from build123d import *

# Parameters (mm, degrees)
CUT_EXTRUDE1_DEPTH      = 136.830777072
CUT_EXTRUDE1_DEPTH_BACK = 136.830777072
SKETCH2_R               = 6
CUT_EXTRUDE2_DEPTH      = 91.967026993
CUT_EXTRUDE2_DEPTH_BACK = 91.967026993
SKETCH4_R               = 2.5


with BuildPart() as part:
    # Sketch1 → Revolve1 (revolve)
    with BuildSketch(Plane(origin=(0, 0, 0), x_dir=(0, 0, -1), z_dir=(1, 0, 0))):
        with BuildLine():
            Line((-42.5, 55), (-42.5, -52.5))
            ThreePointArc((-42.5, -52.5), (-39.571067812, -59.571067812), (-32.5, -62.5))
            Line((-32.5, -62.5), (0, -62.5))
            Line((0, -62.5), (0, -65))
            Line((0, -65), (-35, -65))
            ThreePointArc((-35, -65), (-42.071067812, -62.071067812), (-45, -55))
            Line((-45, -55), (-45, 55))
            Line((-45, 55), (-42.5, 55))
        make_face()
    revolve(axis=Axis((0, 51.85854301, 0), (0, -1, 0)))

    # Sketch2 → Cut-Extrude1 (cut, two sides: drawn at the far end of the back side and taken through both)
    with BuildSketch(Plane.XZ.offset(65).offset(-CUT_EXTRUDE1_DEPTH_BACK)):
        with Locations(Location((0, 12.5, 0), (0, 0, 270))):
            Circle(SKETCH2_R)
        with Locations(Location((0, -12.5, 0), (0, 0, 270))):
            Circle(SKETCH2_R)
    extrude(amount=CUT_EXTRUDE1_DEPTH + CUT_EXTRUDE1_DEPTH_BACK, mode=Mode.SUBTRACT)

    # Sketch4 → Cut-Extrude2 (cut, two sides: drawn at the far end of the back side and taken through both)
    with BuildSketch(Plane.XY.offset(-CUT_EXTRUDE2_DEPTH_BACK)):
        with Locations(Location((0, -5, 0), (0, 0, 180))):
            Circle(SKETCH4_R)
        with Locations(Location((0, -35, 0), (0, 0, 180))):
            Circle(SKETCH4_R)
    extrude(amount=CUT_EXTRUDE2_DEPTH + CUT_EXTRUDE2_DEPTH_BACK, mode=Mode.SUBTRACT)


solid = part.part
Here's how the part is built. I have some questions about the finished solid (model axes, mm). A direction names the side the tool comes from. Give positions to 0.01 mm unless a question says otherwise; leave off trailing zeros. Order: outer loops, then holes, each group sorted by start corner. A loop starts at its lowest first (then second) coordinate and runs counter-clockwise, first axis right, second up. Notation, with made-up numbers: (58.25, 41) -> (77.25, 41) arc R25 cw to (77.25, 73) -> close; hole circle Ø10 at (70, 39). An arc over 180 degrees is marked (long way). Use a Markdown table: item, result. Add a question column.
Item 1: I need wall thicknesses on line 1 (Z direction, x = 0, y = -22); line 2 (Y direction, x = 0, z = -43.8); line 3 (Y direction, x = 0, z = -43.65). Which ranges of each line are inside material? Lowest first, please.
Item 2: If we mould it in two halves opening along Z, with no side actions, what happens to faces 1 (the face through (0.33, -7.48, 43.7)), 2 (the face through (-2.3, -63.73, -18.04)), 3 (the face through (17.235, 0.77, 41.569))? For each: pulls with the +Z half, pulls with the -Z half, needs draft (parallel to the pull), parting line crosses it, or undercut.
Item 3: Imagine slicing it at C-C on y = -47. Please give me the cut outline in (x, z).
Item 4: Imagine slicing it at B-B on z = 0. Please give me the cut outline in (x, y), plus the area to 4 significant figures.
Item 5: Will these pins go through, and if not, where does the flat tip stop? pin 1 (5 mm diameter, centred on x = 10.5, z = -28, fed in from +Y); pin 2 (2 mm diameter, centred on y = -16.5, z = -31, fed in from +X); pin 3 (11 mm diameter, centred on x = 0, z = 12.5, fed in from +Y); pin 4 (5 mm diameter, centred on y = -4.5, z = 21, fed in from +X).
Item 6: For faces 4 (the face through (0.54, -32.56, -43.73)), 5 (the face through (0, -62.5, 0)), which set-ups out of +Z, -Z, +X, -X, +Y, -Y let a thin tool reach every point of the face, with its end or its side?
Data:
| question | item | result |
|---|---|---|
| 1 | line 1 | z = -45 to -42.5, 42.5 to 45 |
| 1 | line 2 | y = -59.75 to -37.5, -32.5 to -7.5, -2.5 to 55 |
| 1 | line 3 | y = -60.02 to -37.5, -32.5 to -7.5, -2.5 to 55 |
| 2 | face 1 | needs draft |
| 2 | face 2 | undercut |
| 2 | face 3 | parting line crosses it |
| 3 | outline | circle Ø90 at (0, 0); hole circle Ø85 at (0, 0) |
| 4 | outline | (-45, -55) arc R10 ccw to (-35, -65) -> (35, -65) arc R10 ccw to (45, -55) -> (45, 55) -> (42.5, 55) -> (42.5, -52.5) arc R10 cw to (32.5, -62.5) -> (-32.5, -62.5) arc R10 cw to (-42.5, -52.5) -> (-42.5, 55) -> (-45, 55) -> close |
| 4 | area | 812.5 mm² |
| 5 | pin 1 | stops at y = -62.5 |
| 5 | pin 2 | stops at x = 33.54 |
| 5 | pin 3 | passes through |
| 5 | pin 4 | stops at x = 41.02 |
| 6 | face 4 | +Z, -Z |
| 6 | face 5 | +Y |
